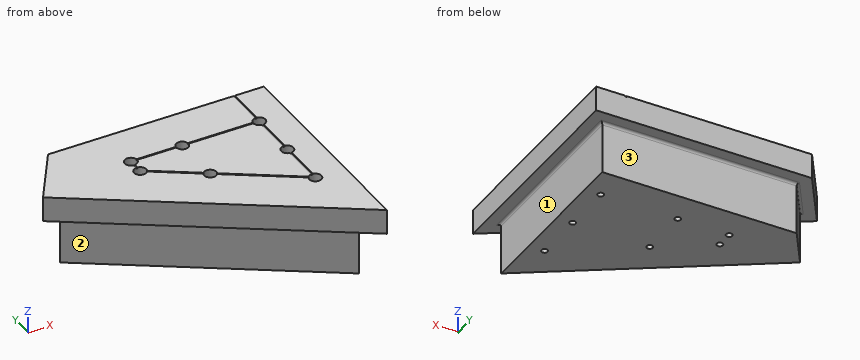
```python
from build123d import *

# Parameters (mm, degrees)
BOSS_EXTRUDE1_DEPTH                             = 70.7898
CBORE_FOR_10_SOCKET_HEAD_CAP_SCREW1_D           = 5.5372
CBORE_FOR_10_SOCKET_HEAD_CAP_SCREW1_CBORE_D     = 11.1252
CBORE_FOR_10_SOCKET_HEAD_CAP_SCREW1_CBORE_DEPTH = 66.8274
BOSS_EXTRUDE2_DEPTH                             = 22.8854
FILLET2_R                                       = 2.3368
CUT_EXTRUDE1_DEPTH                              = 0.762


with BuildPart() as part:
    # Sketch1 → Boss-Extrude1 (new body)
    with BuildSketch(Plane.XY):
        Polygon((-177.8, 0), (-200.472065098, -34.911918701), (0, -165.1), (0, 0), align=None)
    extrude(amount=BOSS_EXTRUDE1_DEPTH)

    # CBORE for #10 Socket Head Cap Screw1 (through all)
    with Locations(Plane.XY.offset(70.7898)):
        with Locations((-132.031708342, -28.575), (-14.535778015, -28.575), (-14.535778015, -74.350066155), (-14.535778015, -120.125132311), (-85.023198604, -74.350066155), (-85.023198604, -28.575), (-132.031708342, -43.822382986)):
            CounterBoreHole(CBORE_FOR_10_SOCKET_HEAD_CAP_SCREW1_D / 2, CBORE_FOR_10_SOCKET_HEAD_CAP_SCREW1_CBORE_D / 2, CBORE_FOR_10_SOCKET_HEAD_CAP_SCREW1_CBORE_DEPTH)

    # Sketch13 → Boss-Extrude2 (add)
    with BuildSketch(Plane.XY.offset(70.7898)):
        Polygon((12.7, 12.7), (-184.695537385, 12.7), (-218.040097055, -38.64611917), (12.7, -188.490490253), align=None)
        Polygon((0, -165.1), (0, 0), (-177.8, 0), (-200.472065098, -34.911918701), align=None, mode=Mode.SUBTRACT)
    extrude(amount=-BOSS_EXTRUDE2_DEPTH)

    # Fillet2
    fillet2_edges = [part.edges().sort_by_distance(p)[0] for p in [
        (-189.136032549, -17.455959351, 47.9044),
        (-100.236032549, -100.005959351, 47.9044),
        (0, -82.55, 47.9044),
        (-88.9, 0, 47.9044),
    ]]
    fillet(fillet2_edges, radius=FILLET2_R)

    # Sketch14 → Cut-Extrude1 (cut)
    with BuildSketch(Plane.XY.offset(70.7898)):
        with BuildLine():
            Line((-14.950792959, -120.764199283), (-132.446723286, -44.461449959))
            ThreePointArc((-132.446723286, -44.461449959), (-132.701366981, -44.185977962), (-132.793708342, -43.822382986))
            Line((-132.793708342, -43.822382986), (-132.793708342, -28.575))
            ThreePointArc((-132.793708342, -28.575), (-132.570523709, -28.036184633), (-132.031708342, -27.813))
            Line((-132.031708342, -27.813), (-15.297778015, -27.813))
            Line((-15.297778015, -27.813), (-15.297778015, 12.7))
            Line((-15.297778015, 12.7), (-13.773778015, 12.7))
            Line((-13.773778015, 12.7), (-13.773778015, -120.125132311))
            ThreePointArc((-13.773778015, -120.125132311), (-14.172183039, -120.79479095), (-14.950792959, -120.764199283))
        make_face()
        with BuildLine():
            Line((-16.474792959, -117.957340453), (-130.922723286, -43.633985473))
            ThreePointArc((-130.922723286, -43.633985473), (-131.177366981, -43.358513475), (-131.269708342, -42.9949185))
            Line((-131.269708342, -42.9949185), (-131.269708342, -30.099))
            ThreePointArc((-131.269708342, -30.099), (-131.046523709, -29.560184633), (-130.507708342, -29.337))
            Line((-130.507708342, -29.337), (-15.297778015, -29.337))
            Line((-15.297778015, -29.337), (-15.297778015, -117.31827348))
            ThreePointArc((-15.297778015, -117.31827348), (-15.696183039, -117.98793212), (-16.474792959, -117.957340453))
        make_face(mode=Mode.SUBTRACT)
    extrude(amount=-CUT_EXTRUDE1_DEPTH, mode=Mode.SUBTRACT)


solid = part.part
```
Verification items for the finished model (mm, model axes). Face numbers are marked on the shaded views. A direction names the side the tool comes from. Coordinates: 2 decimals unless noted, no trailing zeros. Write each loop counter-clockwise with the first axis right and the second up, starting at its lowest first coordinate (ties: lowest second). Pieces come first, ordered by that corner, then holes. Notation, with made-up numbers: M -28,88 L 5,88 A5 cw 5,97 Z; hole C 68,82.5 d6. An arc over 180 degrees is marked long. One line per item, written item: value.
Item 1: Scan lines: line 1 along Y through (x, z) = (-13, 22.5); line 2 along X through (y, z) = (-74, 51); line 3 along X through (y, z) = (-72, 40.5) (3 decimals). Record each from-to range of solid material in increasing order.
Check sheet entries:
line 1: y = -156.66 to -125.47, -114.78 to -79.7, -69 to -33.92, -23.23 to 0
line 2: x = -163.6 to -90.57, -79.47 to -20.09, -8.98 to 12.7
line 3: x = -143.361 to -90.065, -79.981 to -19.578, -9.494 to 0
Item 2: Section check C-C, the plane y = -176. Record the boundary of the cut face in (x, z), plus the area to 3 significant figures.
Check sheet entries:
outline: M -6.53,47.9 L 12.7,47.9 L 12.7,70.79 L -6.53,70.79 Z
area: 440 mm^2
Item 3: Section check B-B, the plane z = 12. Record the boundary of the cut face in (x, y) (3 decimals), plus the area to 3 significant figures.
Check sheet entries:
outline: M -200.472,-34.912 L 0,-165.1 L 0,0 L -177.8,0 Z; hole C -132.032,-43.822 d11.125; hole C -132.032,-28.575 d11.125; hole C -85.023,-74.35 d11.125; hole C -85.023,-28.575 d11.125; hole C -14.536,-120.125 d11.125; hole C -14.536,-74.35 d11.125; hole C -14.536,-28.575 d11.125
area: 19,000 mm^2
Item 4: Gauge pin test, flat ends, axial feed: pin 1 Ø3.5 at (x, y) = (-129.5, -29) entering from +Z; pin 2 Ø23 at (x, z) = (-99.5, 23) entering from +Y; pin 3 Ø12 at (x, z) = (-44.5, 20) entering from -Y; pin 4 Ø3 at (x, y) = (-142.5, -41.5) entering from -Z. Record the tip position at first contact, or that the pin passes through.
Check sheet entries:
pin 1: stops at z = 3.96
pin 2: stops at y = 0
pin 3: stops at y = -140.1
pin 4: stops at z = 0
Item 5: Section check A-A, the plane z = 55.5. Record the boundary of the cut face in (x, y) (1 decimal), plus the area to 3 significant figures.
Check sheet entries:
outline: M -218,-38.6 L 12.7,-188.5 L 12.7,12.7 L -184.7,12.7 Z; hole C -132,-43.8 d11.1; hole C -132,-28.6 d11.1; hole C -85,-74.4 d11.1; hole C -85,-28.6 d11.1; hole C -14.5,-120.1 d11.1; hole C -14.5,-74.4 d11.1; hole C -14.5,-28.6 d11.1
area: 27,600 mm^2
Item 6: Access from +Z, -Z, +X, -X, +Y, -Y to the whole of each face (thin tool, end or side, straight path). Record for the marked faces 1, 2 and 3.
Check sheet entries:
face 1: -Z, +X, +Y, -Y
face 2: -Z, -X, -Y
face 3: -Z, +X, -X, +Y
